The drawing under review shows one solid part. Ordinate dimensions are in mm from its lowest x, y, z. A direction names the side the tool comes from. Coordinates: 2 decimals unless noted, no trailing zeros. Loops run counter-clockwise (first coordinate to the right, second up) from the corner with the lowest first, then second, coordinate; pieces in that order, holes last. Notation, with made-up numbers: M -21,67.5 L -5,67.5 A27 cw -5,106.5 Z; hole C -14,6.5 d3. An arc over 180 degrees is marked long. Use one line per item in the form item = value.
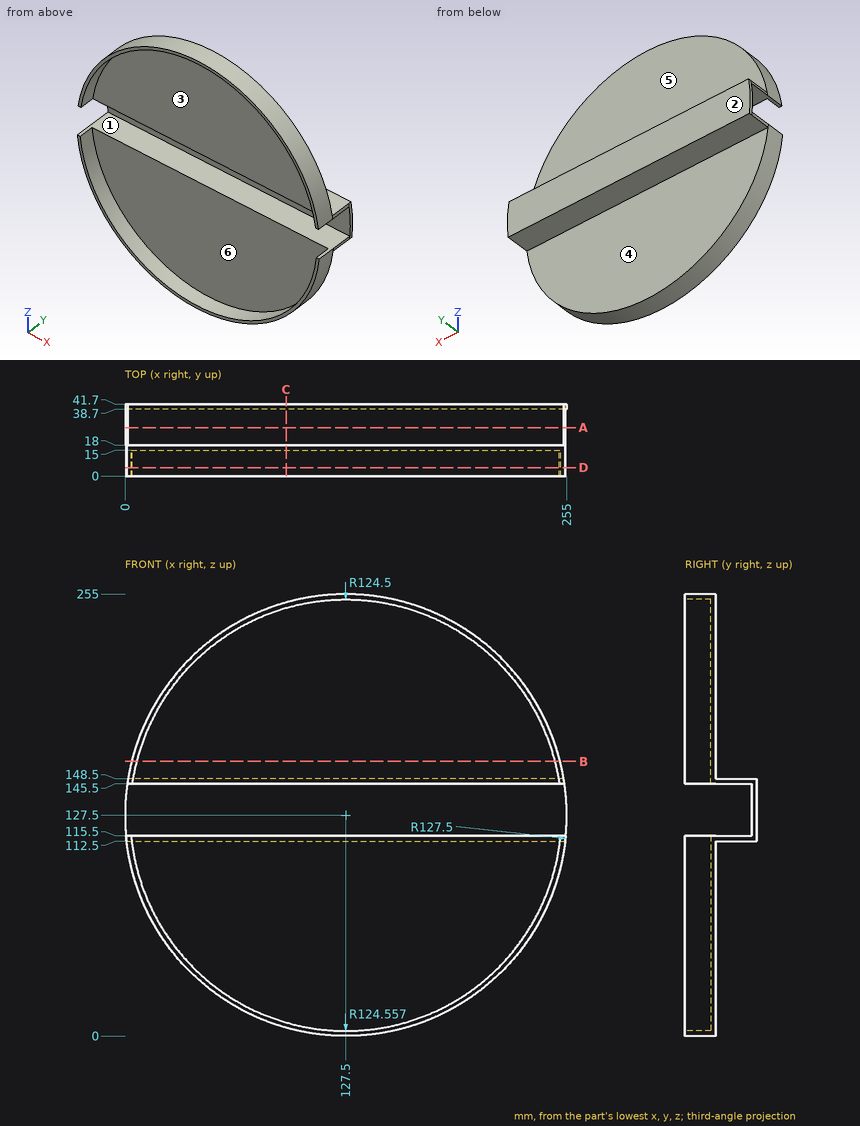
1. For pin 1 Ø7 at (x, y) = (176, 34.5) entering from +Z; pin 2 Ø8 at (x, y) = (96.5, 12) entering from +Z; pin 3 Ø4 at (x, y) = (214.5, 5.5) entering from -Z, all flat-tipped, find the tip position at first contact; note any pin that passes through.
Computed values:
pin_1 = 148.5
pin_2 = 252.11
pin_3 = 32.47
2. Consider section B-B on z = 158.5. Write out the cut boundary in (x, y).
Computed values:
outline = M 3.83,0 L 6.92,0 L 6.92,15 L 248.08,15 L 248.08,0 L 251.17,0 L 251.17,18 L 3.83,18 Z
3. Consider section D-D on y = 5. Write out the cut boundary in (x, z).
Computed values:
outline = M 0.57,115.5 A127.5 ccw 254.43,115.5 L 251.48,115.5 A124.56 cw 3.52,115.5 Z; M 1.28,145.5 L 4.31,145.5 A124.5 cw 250.69,145.5 L 253.72,145.5 A127.5 ccw Z
4. Consider section C-C on x = 93. Write out the cut boundary in (y, z).
Computed values:
outline = M 0,4.76 L 18,4.76 L 18,112.5 L 41.7,112.5 L 41.7,148.5 L 18,148.5 L 18,250.24 L 0,250.24 L 0,247.12 L 15,247.12 L 15,145.5 L 38.7,145.5 L 38.7,115.5 L 15,115.5 L 15,7.82 L 0,7.82 Z
5. Tool access review of the marked faces 1, 2, 3 and 4: name each direction out of +Z, -Z, +X, -X, +Y, -Y from which nothing blocks a thin tool from reaching the whole face with its end or side.
Computed values:
face_1 = +X, -X, -Y
face_2 = +Z, -Z, +X, -X, +Y
face_3 = -Y
face_4 = -Z, +X, -X, +Y
6. Wall thickness on line 1 along Z through (x, y) = (107.5, 33); line 2 along Y through (x, z) = (112, 94.5); line 3 along X through (y, z) = (7, 57) (1 decimal): over which ranges is each line inside the solid? List them lowest first. Write a range as from..to.
Computed values:
line_1 = 112.5..115.5, 145.5..148.5
line_2 = 15..18
line_3 = 21.3..24.8, 230.2..233.7
7. Draft analysis for pull direction X (two halves, no side actions). For the marked faces 5 and 6, state which applies: +X half, -X half, draft (parallel to the pull), parting line (faces both ways), or undercut.
Computed values:
face_5 = draft
face_6 = undercut
8. Consider section A-A on y = 28. Write out the cut boundary in (x, z) (1 decimal), plus the area to 3 significant figures.
Computed values:
outline = M 0.6,115.5 A127.5 ccw 0.9,112.5 L 254.1,112.5 A127.5 ccw 254.4,115.5 Z; M 1.3,145.5 L 253.7,145.5 A127.5 ccw 253.3,148.5 L 1.7,148.5 A127.5 ccw Z
area = 1,520 mm2
